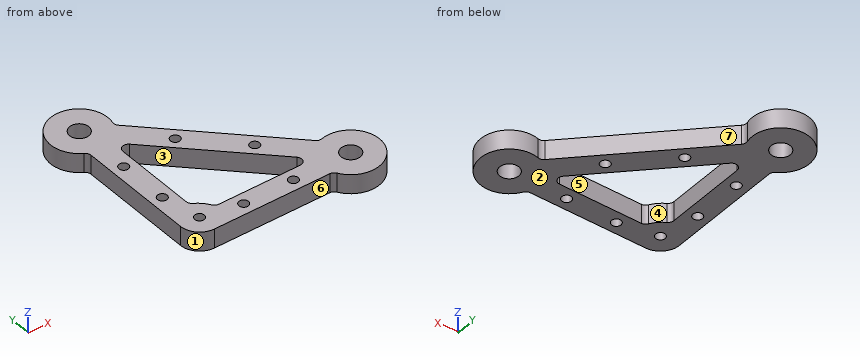
from build123d import *

# Parameters (mm, degrees)
F0_R     = 5
F1_DEPTH = 10
F2_R     = 10
F3_R     = 3
F5_D     = 5


with BuildPart() as f1:
    # F0 (on Top) → F1 (new body)
    with BuildSketch(Plane.XY):
        with BuildLine():
            Line((-6, -6), (66.252273, -6))
            ThreePointArc((66.252273, -6), (93.858193, -5.740251), (74.52153, 13.963752))
            Line((74.52153, 13.963752), (13.963752, 74.52153))
            ThreePointArc((13.963752, 74.52153), (-5.740251, 93.858193), (-6, 66.252273))
            Line((-6, 66.252273), (-6, -6))
        make_face()
        with BuildLine():
            Line((65.514719, 6), (13.747727, 6))
            ThreePointArc((13.747727, 6), (10.606602, 10.606602), (6, 13.747727))
            Line((6, 13.747727), (6, 65.514719))
            Line((6, 65.514719), (65.514719, 6))
        make_face(mode=Mode.SUBTRACT)
        with Locations((80, 0)):
            Circle(F0_R, mode=Mode.SUBTRACT)
        with Locations((0, 80)):
            Circle(F0_R, mode=Mode.SUBTRACT)
    extrude(amount=F1_DEPTH)

    # F2
    f2_edges = [f1.edges().sort_by_distance(p)[0] for p in [
        (-6, -6, 5),
    ]]
    fillet(f2_edges, radius=F2_R)

    # F3
    f3_edges = [f1.edges().sort_by_distance(p)[0] for p in [
        (13.963752, 74.52153, 5),
        (74.52153, 13.963752, 5),
        (66.252273, -6, 5),
        (-6, 66.252273, 5),
        (65.514719, 6, 5),
        (6, 65.514719, 5),
        (6, 13.747727, 5),
        (13.747727, 6, 5),
    ]]
    fillet(f3_edges, radius=F3_R)

    # F5 (through all)
    with Locations(Plane.XY.offset(10)):
        with Locations((0, 50), (0, 24), (28.284271, 51.715729), (51.715729, 28.284271), (50, 0), (24, 0), (4, 4)):
            Hole(F5_D / 2)


solid = f1.part
Check sheet for the modelled part. Datum: model origin and axes. Units: mm. Face numbers are marked on the shaded views. A direction names the side the tool comes from. Round coordinates to 2 decimals unless told otherwise and drop trailing zeros. Order: outer loops, then holes, each group sorted by start corner. A loop starts at its lowest first (then second) coordinate and runs counter-clockwise, first axis right, second up.
(1) Go/stop test with flat-tipped pins: P1, Ø1.5, axis at x = -1.5, z = 7, coming from the +Y side; P2, Ø3, axis at y = 29.5, z = 2.5, coming from the +X side; P3, Ø3, axis at x = 29.5, z = 4.5, coming from the -Y side. Record where each tip stops, or that it passes through.
(2) Scan lines: probe 1 along Y at (x, z) = (0.5, 9); probe 2 along Y at (x, z) = (0, 7.5); probe 3 along Y at (x, z) = (79.5, 7.5). Record each from-to range of solid material in increasing order.
(3) Access from +Z, -Z, +X, -X, +Y, -Y to the whole of each face (thin tool, end or side, straight path). Record for the marked faces 5, 6 and 7.
(4) Cross-section at C-C, the plane z = 3.75. State how many separate pieces and enclosed holes the cut face has, and give its area (3 significant figures).
(5) Draft check along Y on the marked faces 1, 2, 3 and 4. Enter one of: pulls with the +Y half, pulls with the -Y half, needs draft (parallel to the pull), parting line crosses it, or undercut.
(6) Cross-section at A-A, the plane y = 80. Enter the section's corners in (x, z).
Check sheet entries:
1. P1: stops at y = 94.98
1. P2: stops at x = 60.49
1. P3: stops at y = -6
2. probe 1: y = -5.37 to 21.55, 26.45 to 47.55, 52.45 to 75.03, 84.97 to 94.99
2. probe 2: y = -5.17 to 21.5, 26.5 to 47.5, 52.5 to 75, 85 to 95
2. probe 3: y = -14.99 to -4.97, 4.97 to 14.99
3. face 5: +Z, -Z
3. face 6: +Z, -Z, -X, -Y
3. face 7: +Z, -Z, +X, +Y
4. separate pieces: 1
4. enclosed holes: 10
4. area: 3,740 mm2
5. face 1: pulls with the -Y half
5. face 2: needs draft
5. face 3: undercut
5. face 4: undercut
6. outline: (-15, 0) - (-5, 0) - (-5, 10) - (-15, 10) - close; (5, 0) - (15, 0) - (15, 10) - (5, 10) - close
